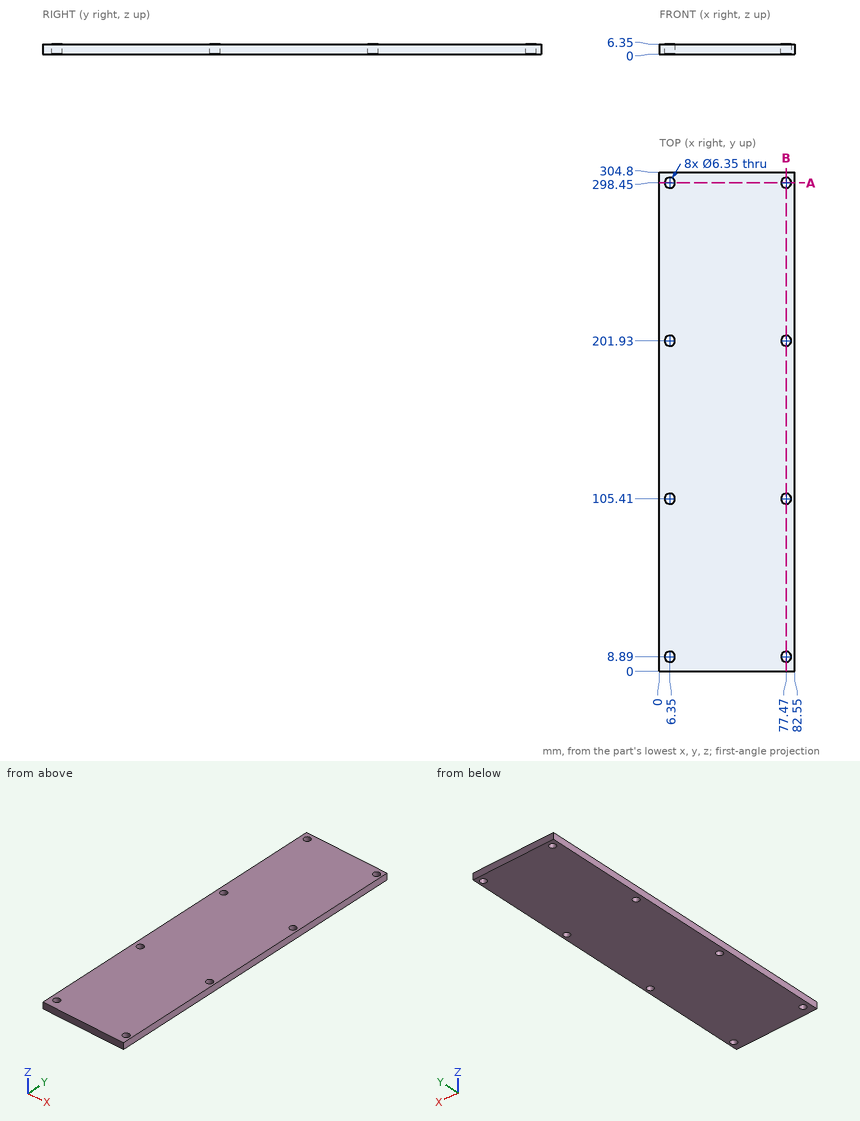
Here's the drawing with two shaded views (mm, measured from the low corner). I have some questions. Give positions to 0.01 mm unless a question says otherwise; leave off trailing zeros. Loops run counter-clockwise (first coordinate to the right, second up) from the corner with the lowest first, then second, coordinate; pieces in that order, holes last. Notation, with made-up numbers: M 20.25,66 L 50.25,66 A12 cw 50.25,80 Z; hole C 13.25,54 d3. An arc over 180 degrees is marked long. One line per item, written item: value. Start each with the question number.
1) If we section it at B-B, the plane x = 77.47: Write out the boundary of the cut face in (y, z) (3 decimals), and give its area (3 significant figures).
2) If I drill on line 1 (X direction, y = 8.89, z = 5) (3 decimals); line 2 (Y direction, x = 6, z = 0.5); line 3 (Y direction, x = 77.47, z = 4.25) (3 decimals), over which ranges is the centre line in solid material (lowest first)? Write a range as [from, to].
3) I'm going to push a flat-ended pin straight in: pin 1 (8.5 mm diameter, centred on x = 6.35, y = 298.45, fed in from +Z). Where does the tip first touch, or does it pass through?
4) If we section it at A-A, the plane y = 298.45: Write out the boundary of the cut face in (x, z) (3 decimals).
Completed:
1. outline: M 0,0 L 5.715,0 L 5.715,6.35 L 0,6.35 Z; M 12.065,0 L 102.235,0 L 102.235,6.35 L 12.065,6.35 Z; M 108.585,0 L 198.755,0 L 198.755,6.35 L 108.585,6.35 Z; M 205.105,0 L 295.275,0 L 295.275,6.35 L 205.105,6.35 Z; M 301.625,0 L 304.8,0 L 304.8,6.35 L 301.625,6.35 Z
1. area: 1,770 mm^2
2. line 1: x = [0, 3.175], [9.525, 74.295], [80.645, 82.55]
2. line 2: y = [0, 5.73], [12.05, 102.25], [108.57, 198.77], [205.09, 295.29], [301.61, 304.8]
2. line 3: y = [0, 5.715], [12.065, 102.235], [108.585, 198.755], [205.105, 295.275], [301.625, 304.8]
3. pin 1: stops at z = 6.35
4. outline: M 0,0 L 3.175,0 L 3.175,6.35 L 0,6.35 Z; M 9.525,0 L 74.295,0 L 74.295,6.35 L 9.525,6.35 Z; M 80.645,0 L 82.55,0 L 82.55,6.35 L 80.645,6.35 Z
